Geometry check sheet. Reference: the model listing, model coordinates, mm. Give positions to 0.01 mm unless a question says otherwise; leave off trailing zeros. Write each loop counter-clockwise with the first axis right and the second up, starting at its lowest first coordinate (ties: lowest second). Pieces come first, ordered by that corner, then holes. Notation, with made-up numbers: (48.25, 10.5) - (94.25, 10.5) arc R28 cw to (94.25, 43.5) - close; hole circle Ø11 at (81.25, 35). An arc over 180 degrees is marked (long way). Use a Markdown table: item, result.
```python
from build123d import *

# Parameters (mm, degrees)
ESQUISSE2_R        = 11
ESQUISSE2_R_2      = 8.5
ESQUISSE3_R        = 11
ESQUISSE3_R_2      = 8.5
BOSS_EXTRU_1_DEPTH = 102
ESQUISSE4_R        = 11
ESQUISSE4_R_2      = 8.5
BOSS_EXTRU_2_DEPTH = 96


with BuildPart() as part:
    # Base-Balayage: sweep along a path in Esquisse1
    with BuildLine(Plane.XY) as base_balayage_path:
        ThreePointArc((-65.817930688, 38), (-65.817930688, -38), (0, -76))
    # Esquisse2 → Base-Balayage (sweep)
    with BuildSketch(Plane(origin=(0, 0, 0), x_dir=(0, 0, -1), z_dir=(1, 0, 0))):
        with Locations((0, -76)):
            Circle(ESQUISSE2_R)
        with Locations((0, -76)):
            Circle(ESQUISSE2_R_2, mode=Mode.SUBTRACT)
    sweep(path=base_balayage_path.line)

    # Esquisse3 → Boss.-Extru.1 (add)
    with BuildSketch(Plane(origin=(0, 0, 0), x_dir=(0, 0, -1), z_dir=(1, 0, 0))):
        with Locations(Location((0, -76, 0), (0, 0, 270))):
            Circle(ESQUISSE3_R)
        with Locations(Location((0, -76, 0), (0, 0, 270))):
            Circle(ESQUISSE3_R_2, mode=Mode.SUBTRACT)
    extrude(amount=BOSS_EXTRU_1_DEPTH)

    # Esquisse4 → Boss.-Extru.2 (add)
    with BuildSketch(Plane(origin=(0, 0, 0), x_dir=(-0.8660254037844417, 0.4999999999999947, 0), z_dir=(0.49999999999999484, 0.8660254037844418, 0))):
        with Locations((76, 0)):
            Circle(ESQUISSE4_R)
        with Locations((76, 0)):
            Circle(ESQUISSE4_R_2, mode=Mode.SUBTRACT)
    extrude(amount=BOSS_EXTRU_2_DEPTH)


solid = part.part
```
1) Mould release check, pull along Y, two halves, no side actions. Record for faces 1 (the cylindrical face through (50, -65, 0)), 2 (the cylindrical face through (50.29, -67.51, -0.37)), 3 (the cylindrical face through (-40.09, 77.79, -10.74)), 4 (the flat face through (102, -79.2, 8.1)): pulls with the +Y half, pulls with the -Y half, needs draft (parallel to the pull), parting line crosses it, or undercut.
Working result:
| item | result |
|---|---|
| face 1 | parting line crosses it |
| face 2 | undercut |
| face 3 | undercut |
| face 4 | needs draft |
2) Section check C-C on x = -14. Count the separate pieces of the cut face and the enclosed holes in it, then the cut area to 3 significant figures.
Working result:
| item | result |
|---|---|
| separate pieces | 2 |
| enclosed holes | 1 |
| area | 263 mm² |
3) Section check B-B on x = 31. Record the boundary of the cut face in (y, z), then the cut area to 3 significant figures.
Working result:
| item | result |
|---|---|
| outline | circle Ø22 at (-76, 0); hole circle Ø17 at (-76, 0) |
| area | 153 mm² |
4) Section check A-A on z = 0. Record the boundary of the cut face in (x, y).
Working result:
| item | result |
|---|---|
| outline | (-75.34, 43.5) arc R87 ccw to (0, -87) - (102, -87) - (102, -84.5) - (0, -84.5) arc R84.5 cw to (-73.18, 42.25) - (-25.18, 125.39) - (-27.34, 126.64) - close; (-58.46, 33.75) arc R67.5 ccw to (0, -67.5) - (102, -67.5) - (102, -65) - (0, -65) arc R65 cw to (-56.29, 32.5) - (-8.29, 115.64) - (-10.46, 116.89) - close |
5) Depth check by flat-ended pin: P1, Ø2, axis at x = 67, z = 6.5, coming from the -Y side; P2, Ø10, axis at x = -37, y = -54.5, coming from the -Z side; P3, Ø3, axis at y = -18, z = 9, coming from the +X side. Enter the tip coordinate at first touch or a pass-through.
Working result:
| item | result |
|---|---|
| P1 | stops at y = -85.53 |
| P2 | stops at z = -9.73 |
| P3 | stops at x = -65.47 |
6) Material ranges on L1, parallel to Z at x = 76.5, y = -76; L2, parallel to Y at x = -53.5, z = -4.75; L3, parallel to Y at x = -43, z = -0.75, recorded low to high. Write a range as from..to.
Working result:
| item | result |
|---|---|
| L1 | z = -11..-8.5, 8.5..11 |
| L2 | y = -67.23..-63.52, -43.5..-38.78, 39.49..45.24, 73.43..79.18 |
| L3 | y = -75.6..-72.7, -52.07..-48.78, 55.57..60.59, 94.46..99.47 |
